Here's how the part is built. I have some questions about the finished solid (model axes, mm). A direction names the side the tool comes from. Coordinates: 2 decimals unless noted, no trailing zeros. Write each loop counter-clockwise with the first axis right and the second up, starting at its lowest first coordinate (ties: lowest second). Pieces come first, ordered by that corner, then holes. Notation, with made-up numbers: M 58,36 L 70,36 A9 ccw 70,47 Z; hole C 11,80 d2. An arc over 180 degrees is marked long. Use one line per item in the form item = value. Start each with the question number.
1. On a 3-axis mill with a long thin cutter (end or side, diameter ignored), from which of +Z, -Z, +X, -X, +Y, -Y can I reach the whole of each face in a straight line? I mean faces 1 (the face through (-1.136, -0.019, 37.869)), 2 (the face through (-0.083, 1.878, -2.045)). Say none if no direction works.
2. I want a section at A-A, the plane z = -23. List the corners of the cut face in (x, y) for me, plus the area to 3 significant figures.
3. Please list where these lines run through material, in increasing order: line 1 along Z through (x, y) = (-2.75, -0.75) (3 decimals); line 2 along X through (y, z) = (-0.5, -24); line 3 along Y through (x, z) = (0, -5). Write a range as [from, to].
4. I'm going to push flat-ended pins straight in: pin 1 Ø4 at (y, z) = (-2, -23.5) entering from -X; pin 2 Ø3 at (y, z) = (3, 16.5) entering from -X. Where does each tip first touch, or does it pass through?
from build123d import *

# Parameters (mm, degrees)
CUT_EXTRUDE1_DEPTH      = 42.360505525
CIRPATTERN1_COUNT       = 4
SKETCH5_W               = 0.79375
SKETCH5_H               = 3.96875
FILLET1_R               = 0.18796
CUT_EXTRUDE3_REACH      = 43.876
CUT_EXTRUDE3_END_RADIUS = 1.8161
SKETCH6_W               = 0.3175
SKETCH6_H               = 2.3495


with BuildPart() as part:
    # Sketch2 → Revolve1 (revolve)
    with BuildSketch(Plane(origin=(0, 0, 0), x_dir=(0, 0, -1), z_dir=(1, 0, 0))):
        Polygon((-35.6362, -1.8796), (41.275, -1.8796), (41.275, 0), (-41.275, 0), (-41.275, -1.8796), align=None)
    revolve(axis=Axis((0, 0, 41.275), (0, 0, -1)))

    # Sketch3 → Cut-Extrude1 (cut, symmetric)
    with BuildSketch(Plane(origin=(0, 0, 0), x_dir=(0, 0, -1), z_dir=(1, 0, 0))):
        Polygon((-41.275, -0.00254), (-35.6362, -1.8796), (-41.275, -1.8796), align=None)
    cut_extrude1 = extrude(amount=CUT_EXTRUDE1_DEPTH, both=True, mode=Mode.SUBTRACT)

    # CirPattern1: Cut-Extrude1 ×4 about axis
    cirpattern1_axis = Axis((0, 0, 0), (0, 0, 1))
    for i in range(1, CIRPATTERN1_COUNT):
        add(cut_extrude1.rotate(cirpattern1_axis, i * 360 / CIRPATTERN1_COUNT), mode=Mode.SUBTRACT)

    # Sketch5 → Revolve2 (revolve)
    with BuildSketch(Plane(origin=(0, 0, 0), x_dir=(0, 0, -1), z_dir=(1, 0, 0)), mode=Mode.PRIVATE) as revolve2_sk:
        with Locations((40.878125, 1.984375)):
            Rectangle(SKETCH5_W, SKETCH5_H)
    revolve(revolve2_sk.sketch.rotate(Axis((0, 0, -41.275), (0, 0, 1)), 135), axis=Axis((0, 0, -41.275), (0, 0, 1)))

    # Fillet1
    fillet1_edges = [part.edges().sort_by_distance(p)[0] for p in [
        (0, 1.8796, -40.48125),
    ]]
    fillet(fillet1_edges, radius=FILLET1_R)

    # Cut-Extrude3: up to this cylinder (the profile starts outside it)
    cut_extrude3_end = Plane(origin=(0, 0, -35.56), z_dir=(0, 0, 1)) * Cylinder(CUT_EXTRUDE3_END_RADIUS, 96.8292, mode=Mode.PRIVATE)
    # Sketch6 → Cut-Extrude3 (cut, up to the surface)
    with BuildSketch(Plane(origin=(1.8796, 0, 0), x_dir=(0, 0, -1), z_dir=(1, 0, 0)), mode=Mode.PRIVATE) as cut_extrude3_sk1:
        with Locations((33.3375, 0)):
            Rectangle(SKETCH6_W, SKETCH6_H)
    cut_extrude3_tool1 = extrude(cut_extrude3_sk1.sketch, amount=-CUT_EXTRUDE3_REACH, mode=Mode.PRIVATE) - cut_extrude3_end
    # Sketch6 → Cut-Extrude3 (cut, up to the surface)
    with BuildSketch(Plane(origin=(1.8796, 0, 0), x_dir=(0, 0, -1), z_dir=(1, 0, 0)), mode=Mode.PRIVATE) as cut_extrude3_sk2:
        with Locations((34.44875, 0)):
            Rectangle(SKETCH6_W, SKETCH6_H)
    cut_extrude3_tool2 = extrude(cut_extrude3_sk2.sketch, amount=-CUT_EXTRUDE3_REACH, mode=Mode.PRIVATE) - cut_extrude3_end
    # Sketch6 → Cut-Extrude3 (cut, up to the surface)
    with BuildSketch(Plane(origin=(1.8796, 0, 0), x_dir=(0, 0, -1), z_dir=(1, 0, 0)), mode=Mode.PRIVATE) as cut_extrude3_sk3:
        with Locations((35.56, 0)):
            Rectangle(SKETCH6_W, SKETCH6_H)
    cut_extrude3_tool3 = extrude(cut_extrude3_sk3.sketch, amount=-CUT_EXTRUDE3_REACH, mode=Mode.PRIVATE) - cut_extrude3_end
    # Sketch6 → Cut-Extrude3 (cut, up to the surface)
    with BuildSketch(Plane(origin=(1.8796, 0, 0), x_dir=(0, 0, -1), z_dir=(1, 0, 0)), mode=Mode.PRIVATE) as cut_extrude3_sk4:
        with Locations((36.67125, 0)):
            Rectangle(SKETCH6_W, SKETCH6_H)
    cut_extrude3_tool4 = extrude(cut_extrude3_sk4.sketch, amount=-CUT_EXTRUDE3_REACH, mode=Mode.PRIVATE) - cut_extrude3_end
    # Sketch6 → Cut-Extrude3 (cut, up to the surface)
    with BuildSketch(Plane(origin=(1.8796, 0, 0), x_dir=(0, 0, -1), z_dir=(1, 0, 0)), mode=Mode.PRIVATE) as cut_extrude3_sk5:
        with Locations((37.7825, 0)):
            Rectangle(SKETCH6_W, SKETCH6_H)
    cut_extrude3_tool5 = extrude(cut_extrude3_sk5.sketch, amount=-CUT_EXTRUDE3_REACH, mode=Mode.PRIVATE) - cut_extrude3_end
    cut_extrude3 = cut_extrude3_tool1.solids().sort_by_distance((1.8796, 0, -33.3375))[0] + cut_extrude3_tool2.solids().sort_by_distance((1.8796, 0, -34.44875))[0] + cut_extrude3_tool3.solids().sort_by_distance((1.8796, 0, -35.56))[0] + cut_extrude3_tool4.solids().sort_by_distance((1.8796, 0, -36.67125))[0] + cut_extrude3_tool5.solids().sort_by_distance((1.8796, 0, -37.7825))[0]
    add(cut_extrude3, mode=Mode.SUBTRACT)

    # Mirror1: Cut-Extrude3 across plane
    add(cut_extrude3.mirror(Plane(origin=(0, 0, 0), x_dir=(0, 0, 1), z_dir=(1, 0, 0))), mode=Mode.SUBTRACT)


solid = part.part
Answer list:
q1.face_1 = +Z, -X, +Y, -Y
q1.face_2 = +Z
q2.outline = C 0,0 d3.76
q2.area = 11.1 mm²
q3.line_1 = [-41.275, -40.481]
q3.line_2 = [-1.81, 1.81]
q3.line_3 = [-1.88, 1.88]
q4.pin_1 = -1.88
q4.pin_2 = -1.13
